from build123d import *

# Parameters (mm, degrees)
SKETCH1_W                                      = 54.161
SKETCH1_H                                      = 30
BOSS_EXTRUDE1_DEPTH                            = 5
M4_CLEARANCE_HOLE1_D                           = 4.7
FILLET1_R                                      = 1
CBORE_FOR_6_SOCKET_HEAD_CAP_SCREW1_D           = 3.7973
CBORE_FOR_6_SOCKET_HEAD_CAP_SCREW1_CBORE_D     = 7.14502
CBORE_FOR_6_SOCKET_HEAD_CAP_SCREW1_CBORE_DEPTH = 3.5052


with BuildPart() as part:
    # Sketch1 → Boss-Extrude1 (new body)
    with BuildSketch(Plane.XY):
        with Locations((27.0805, 15)):
            Rectangle(SKETCH1_W, SKETCH1_H)
    extrude(amount=BOSS_EXTRUDE1_DEPTH)

    # M4 Clearance Hole1 (through all)
    with Locations(Plane.XY.offset(5)):
        with Locations((4, 20), (50.161, 20)):
            Hole(M4_CLEARANCE_HOLE1_D / 2)

    # Fillet1
    fillet1_edges = [part.edges().sort_by_distance(p)[0] for p in [
        (0, 30, 2.5),
        (54.161, 30, 2.5),
        (54.161, 0, 2.5),
        (0, 0, 2.5),
    ]]
    fillet(fillet1_edges, radius=FILLET1_R)

    # CBORE for #6 Socket Head Cap Screw1 (through all)
    with Locations(Plane(origin=(0, 0, 0), x_dir=(-1, 0, 0), z_dir=(0, 0, -1))):
        with Locations((-40.986, 24.779), (-13.175, 24.779), (-40.986, 5.221), (-13.175, 5.221)):
            CounterBoreHole(CBORE_FOR_6_SOCKET_HEAD_CAP_SCREW1_D / 2, CBORE_FOR_6_SOCKET_HEAD_CAP_SCREW1_CBORE_D / 2, CBORE_FOR_6_SOCKET_HEAD_CAP_SCREW1_CBORE_DEPTH)


solid = part.part
Can you work these out from the model? Positions are in its coordinate system, mm. A direction names the side the tool comes from. Coordinates: 2 decimals unless noted, no trailing zeros. Loops run counter-clockwise (first coordinate to the right, second up) from the corner with the lowest first, then second, coordinate; pieces in that order, holes last. Notation, with made-up numbers: (-32, 12.25) - (-27, 12.25) arc R37 cw to (-27, 49.25) - close; hole circle Ø4 at (-26.75, 17). An arc over 180 degrees is marked (long way). Put each result on its own line as item: value. Start each with the question number.
Item 1: Suppose I cut it at C-C (z = 4.1). Please give me the cut outline in (x, y) (3 decimals), and give its area (3 significant figures).
Item 2: Which directions (+Z, -Z, +X, -X, +Y, -Y) give clear straight access to the entire face, cutting with the end or side of a thin tool? Please do faces 1 (the face through (2.916, 17.915, 2.465)), 2 (the face through (39, 23, 3.505)).
Item 3: Suppose I cut it at D-D (y = 27.25). Please give me the cut outline in (x, z).
Item 4: If I drill on line 1 along X through (y, z) = (5.5, 1.8); line 2 along X through (y, z) = (26.5, 1.3); line 3 along Y through (x, z) = (4, 1.9), over which ranges is the centre line in solid material (lowest first)?
Item 5: For pin 1 (8 mm diameter, centred on x = 13.175, y = 5.221, fed in from -Z); pin 2 (2 mm diameter, centred on x = 40.5, y = 26, fed in from -Z); pin 3 (3 mm diameter, centred on x = 50.161, y = 20, fed in from +Z), each with a flat end and sliding along its axis, tell me the tip position at first contact or that it passes through.
Item 6: Suppose I cut it at B-B (x = 4). Please give me the cut outline in (y, z).
Item 7: Suppose I cut it at A-A (y = 20). Please give me the cut outline in (x, z), and give its area (3 significant figures).
Item 8: If we mould it in two halves opening along X, with no side actions, what happens to faces 3 (the face through (27, 30, 2)), 4 (the face through (53.86, 0.285, 2.535)), 5 (the face through (39.34, 21.61, 1.73))? For each: +X half, -X half, draft (parallel to the pull), parting line (faces both ways), or undercut.
Here are the results:
1. outline: (0, 1) arc R1 ccw to (1, 0) - (53.161, 0) arc R1 ccw to (54.161, 1) - (54.161, 29) arc R1 ccw to (53.161, 30) - (1, 30) arc R1 ccw to (0, 29) - close; hole circle Ø4.7 at (4, 20); hole circle Ø3.797 at (13.175, 5.221); hole circle Ø3.797 at (13.175, 24.779); hole circle Ø3.797 at (40.986, 5.221); hole circle Ø3.797 at (40.986, 24.779); hole circle Ø4.7 at (50.161, 20)
1. area: 1,540 mm²
2. face 1: +Z, -Z
2. face 2: -Z
3. outline: (0, 0) - (10.59, 0) - (10.59, 3.51) - (15.76, 3.51) - (15.76, 0) - (38.41, 0) - (38.41, 3.51) - (43.57, 3.51) - (43.57, 0) - (54.16, 0) - (54.16, 5) - (0, 5) - close
4. line 1: 0 to 9.61, 16.74 to 37.42, 44.55 to 54.16
4. line 2: 0 to 10.04, 16.31 to 37.86, 44.12 to 54.16
4. line 3: 0 to 17.65, 22.35 to 30
5. pin 1: z = 0
5. pin 2: z = 3.51
5. pin 3: through
6. outline: (0, 0) - (17.65, 0) - (17.65, 5) - (0, 5) - close; (22.35, 0) - (30, 0) - (30, 5) - (22.35, 5) - close
7. outline: (0, 0) - (1.65, 0) - (1.65, 5) - (0, 5) - close; (6.35, 0) - (47.81, 0) - (47.81, 5) - (6.35, 5) - close; (52.51, 0) - (54.16, 0) - (54.16, 5) - (52.51, 5) - close
7. area: 224 mm²
8. face 3: draft
8. face 4: +X half
8. face 5: undercut
